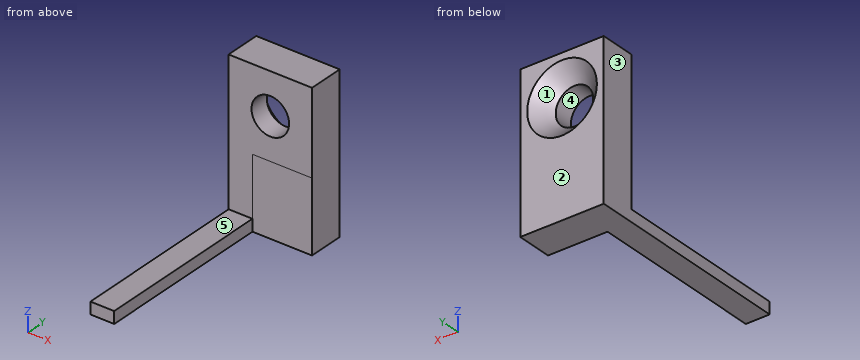
```python
from build123d import *

# Parameters (mm, degrees)
PAD_DEPTH        = 7
SKETCH001_W      = 12.044716
SKETCH001_H      = 19.424721
POCKET_DEPTH     = 6.001
HOLE_D           = 3.15
HOLE_CSINK_D     = 5.85
HOLE_CSINK_ANGLE = 90


with BuildPart() as part:
    # Sketch → Pad (new body)
    with BuildSketch(Plane.YZ):
        Polygon((0, 7), (0, -5), (-15, -5), (-15, -6), (3, -6), (3, 7), align=None)
    extrude(amount=PAD_DEPTH)

    # Sketch001 → Pocket (cut, through all)
    with BuildSketch(Plane.XY):
        with Locations((8.022358, -9.71236)):
            Rectangle(SKETCH001_W, SKETCH001_H)
    extrude(amount=-POCKET_DEPTH, mode=Mode.SUBTRACT)

    # Hole (through all)
    with Locations(Plane(origin=(0, 3, 0), x_dir=(1, 0, 0), z_dir=(0, 1, 0))):
        with Locations((3.5, -3.5)):
            CounterSinkHole(HOLE_D / 2, HOLE_CSINK_D / 2, counter_sink_angle=HOLE_CSINK_ANGLE)


solid = part.part
```
Could you check a few things on this model? Use its own coordinates, in mm. Face numbers are marked on the shaded views. A direction names the side the tool comes from. Round coordinates to 2 decimals unless told otherwise and drop trailing zeros. Loops run counter-clockwise (first coordinate to the right, second up) from the corner with the lowest first, then second, coordinate; pieces in that order, holes last. Notation, with made-up numbers: (86.25, -11.5) - (120.25, -11.5) arc R19 cw to (120.25, 18.5) - close; hole circle Ø10 at (67.5, 70.25). An arc over 180 degrees is marked (long way). Answer as CSV lines item,"result".
1. I want a section at A-A on z = 3.5. List the corners of the cut face in (x, y) for me (3 decimals).
Filled in:
outline,"(0, 0) - (1.925, 0) - (1.925, 1.65) - (0.575, 3) - (0, 3) - close; (5.075, 0) - (7, 0) - (7, 3) - (6.425, 3) - (5.075, 1.65) - close"
2. I want a section at B-B on x = 3.5. List the corners of the cut face in (y, z) for me (3 decimals).
Filled in:
outline,"(0, -6) - (3, -6) - (3, 0.575) - (1.65, 1.925) - (0, 1.925) - close; (0, 5.075) - (1.65, 5.075) - (3, 6.425) - (3, 7) - (0, 7) - close"
3. I want a section at C-C on y = -12.5. List the corners of the cut face in (x, z) for me.
Filled in:
outline,"(0, -6) - (2, -6) - (2, -5) - (0, -5) - close"
4. Please list where these lines run through material, in increasing order: line 1 along Z through (x, y) = (3.5, 1) (3 decimals); line 2 along Y through (x, z) = (1.25, -4.25); line 3 along Z through (x, y) = (0.5, -10.25). Write a range as [from, to].
Filled in:
line 1,"z = [-6, 1.925], [5.075, 7]"
line 2,"y = [0, 3]"
line 3,"z = [-6, -5]"
5. We'd pull the mould along X, two halves only. Please class the marked faces 1, 2 and 3: +X half, -X half, draft (parallel to the pull), parting line (faces both ways), or undercut.
Filled in:
face 1,"undercut"
face 2,"draft"
face 3,"-X half"
6. On a 3-axis mill with a long thin cutter (end or side, diameter ignored), from which of +Z, -Z, +X, -X, +Y, -Y can I reach the whole of each face in a straight line? I mean the marked faces 4 and 5. Say none if no direction works.
Filled in:
face 4,"+Y, -Y"
face 5,"+Z, +X, -X, -Y"
7. For pin 1 Ø3 at (y, z) = (-5.5, -4) entering from +X; pin 2 Ø1 at (x, y) = (0.5, -7.5) entering from +Z; pin 3 Ø3 at (x, z) = (2.5, 5.5) entering from -Y, each with a flat end and sliding along its axis, tell me the tip position at first contact or that it passes through.
Filled in:
pin 1,"stops at x = 2"
pin 2,"stops at z = -5"
pin 3,"stops at y = 0"
8. I want a section at D-D on z = -3.5. List the corners of the cut face in (x, y) for me, then the cut area to 3 significant figures.
Filled in:
outline,"(0, 0) - (7, 0) - (7, 3) - (0, 3) - close"
area,"21.0 mm^2"
